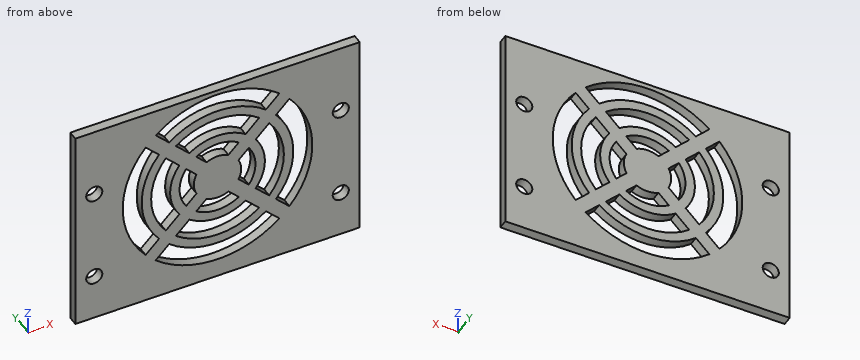
from build123d import *

# Parameters (mm, degrees)
SKETCH1_W                  = 60
SKETCH1_H                  = 45
BOSS_EXTRUDE1_DEPTH        = 2
F_3_4_3_4_DIAMETER_HOLE1_D = 3.4
SKETCH5_R                  = 2.5
AIR_HOLES_DEPTH            = 76.026661928
CIRPATTERN1_COUNT          = 4
SKETCH6_R                  = 2.5
BOSS_EXTRUDE3_DEPTH        = 2


with BuildPart() as part:
    # Sketch1 → Boss-Extrude1 (new body)
    with BuildSketch(Plane(origin=(0, 0, 0), x_dir=(1, 0, 0), z_dir=(0, 1, 0))):
        with Locations((30, 22.5)):
            Rectangle(SKETCH1_W, SKETCH1_H)
    extrude(amount=BOSS_EXTRUDE1_DEPTH)

    # Ø3.4 (3.4) Diameter Hole1 (through all)
    with Locations(Plane(origin=(0, 2, 0), x_dir=(1, 0, 0), z_dir=(0, 1, 0))):
        with Locations((4, 15), (4, 35), (56, 35), (56, 15)):
            Hole(F_3_4_3_4_DIAMETER_HOLE1_D / 2)

    # Sketch5 → Air holes (cut, through all)
    with BuildSketch(Plane(origin=(0, 2, 0), x_dir=(1, 0, 0), z_dir=(0, 1, 0))):
        with Locations(Location((30, 21, 0), (0, 0, 270))):
            Circle(SKETCH5_R)
        with BuildLine():
            Line((21.218150329, 31.903170014), (24.069594445, 29.051725899))
            ThreePointArc((24.069594445, 29.051725899), (30, 31), (35.930405555, 29.051725899))
            Line((35.930405555, 29.051725899), (38.781849671, 31.903170014))
            ThreePointArc((38.781849671, 31.903170014), (30, 35), (21.218150329, 31.903170014))
        make_face()
        with BuildLine():
            Line((25.504132479, 27.617187865), (27.687975781, 25.433344563))
            ThreePointArc((27.687975781, 25.433344563), (30, 26), (32.312024219, 25.433344563))
            Line((32.312024219, 25.433344563), (34.495867521, 27.617187865))
            ThreePointArc((34.495867521, 27.617187865), (30, 29), (25.504132479, 27.617187865))
        make_face()
        with BuildLine():
            Line((40.203220154, 33.324540498), (43.041644604, 36.162964948))
            ThreePointArc((43.041644604, 36.162964948), (30, 41), (16.958355396, 36.162964948))
            Line((16.958355396, 36.162964948), (19.796779846, 33.324540498))
            ThreePointArc((19.796779846, 33.324540498), (30, 37), (40.203220154, 33.324540498))
        make_face()
    air_holes = extrude(amount=-AIR_HOLES_DEPTH, mode=Mode.SUBTRACT)

    # CirPattern1: Air holes ×4 about axis
    cirpattern1_axis = Axis((30, 0, -21), (0, 1, 0))
    for i in range(1, CIRPATTERN1_COUNT):
        add(air_holes.rotate(cirpattern1_axis, i * 360 / CIRPATTERN1_COUNT), mode=Mode.SUBTRACT)

    # Sketch6 → Boss-Extrude3 (add)
    with BuildSketch(Plane(origin=(0, 2, 0), x_dir=(1, 0, 0), z_dir=(0, 1, 0))):
        with Locations((30, 21)):
            Circle(SKETCH6_R)
    extrude(amount=-BOSS_EXTRUDE3_DEPTH)


solid = part.part
Model file for the job. Use its own axes, mm. Give positions to 0.01 mm unless a question says otherwise; leave off trailing zeros. Order: outer loops, then holes, each group sorted by start corner. A loop starts at its lowest first (then second) coordinate and runs counter-clockwise, first axis right, second up. Notation, with made-up numbers: (13.25, 57) - (17.25, 57) arc R12 ccw to (17.25, 72) - close; hole circle Ø1 at (44.5, -34.75). An arc over 180 degrees is marked (long way). Write item = value, one per line. Start each with the question number.
1. Cut at A-A, the plane z = -17.5. List the corners of the cut face in (x, y).
2. Drop a flat-ended pin along its axis: P1, Ø3, axis at x = 4, z = -35, coming from the +Y side. Give the stop position or say it passes through.
3. Cut at C-C, the plane x = 12. List the corners of the cut face in (y, z).
4. Cut at D-D, the plane y = 0.85. State how many separate pieces and enclosed holes the cut face has, and give its area (3 significant figures).
5. Probe line 1 along Z through (x, y) = (4, 1.5); line 2 along X through (y, z) = (0.4, -12); line 3 along X through (y, z) = (0.5, -10). List the from-to ranges inside material, lowest first.
6. Cut at B-B, the plane x = 4. List the corners of the cut face in (y, z).
Taken from the geometry:
q1.outline = (0, 0) - (10.31, 0) - (10.31, 2) - (0, 2) - close; (14.39, 0) - (16.44, 0) - (16.44, 2) - (14.39, 2) - close; (20.63, 0) - (22.81, 0) - (22.81, 2) - (20.63, 2) - close; (24.38, 0) - (35.62, 0) - (35.62, 2) - (24.38, 2) - close; (37.19, 0) - (39.37, 0) - (39.37, 2) - (37.19, 2) - close; (43.56, 0) - (45.61, 0) - (45.61, 2) - (43.56, 2) - close; (49.69, 0) - (60, 0) - (60, 2) - (49.69, 2) - close
q2.P1 = through
q3.outline = (0, -45) - (2, -45) - (2, -29.72) - (0, -29.72) - close; (0, -12.28) - (2, -12.28) - (2, 0) - (0, 0) - close
q4.separate_pieces = 1
q4.enclosed_holes = 16
q4.area = 1,920 mm²
q5.line_1 = -45 to -36.7, -33.3 to -16.7, -13.3 to 0
q5.line_2 = 0 to 12.14, 16.77 to 23.12, 25.64 to 34.36, 36.88 to 43.23, 47.86 to 60
q5.line_3 = 0 to 13.3, 16.88 to 21.34, 38.66 to 43.12, 46.7 to 60
q6.outline = (0, -45) - (2, -45) - (2, -36.7) - (0, -36.7) - close; (0, -33.3) - (2, -33.3) - (2, -16.7) - (0, -16.7) - close; (0, -13.3) - (2, -13.3) - (2, 0) - (0, 0) - close
